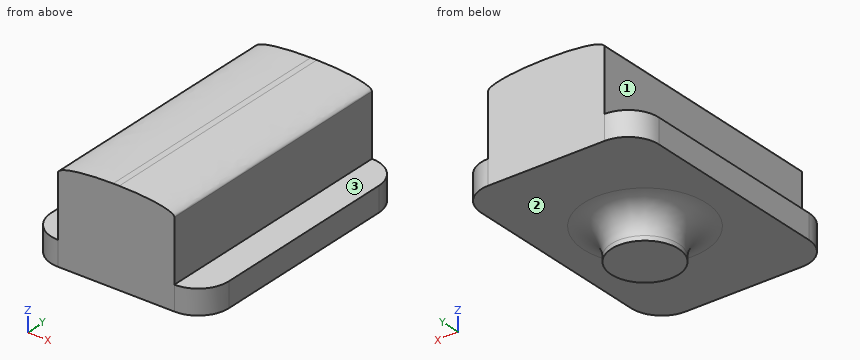
```python
from build123d import *

# Parameters (mm, degrees)
EXTRUDE_1_DEPTH          = 3.1
EXTRUDE_2_DEPTH          = 0.8
FILLET_1_SIZE            = 0.3
FILLET_1_SIZE_2          = 1.8
SKETCH_3_R               = 1
SKETCH_3_R_2             = 1.096749421
EXTRUDE_3_DEPTH          = 1.05
FILLET_5_R               = 0.9
CUT_EXTRUDE_2_DEPTH      = 82.307539193
CUT_EXTRUDE_2_DEPTH_BACK = 82.307539193
SKETCH_7_W               = 25.8
SKETCH_7_H               = 28.300000874
SKETCH_7_W_2             = 5.8
SKETCH_7_H_2             = 8.300000874
FILLET_6_R               = 1


with BuildPart() as part:
    # 草图1 → 凸台-拉伸1 (new body)
    with BuildSketch(Plane.XY):
        with BuildLine():
            Line((-1.3, -78.273), (-1.3, -61.672998253))
            ThreePointArc((-1.3, -61.672998253), (0.6, -59.772998253), (2.5, -61.672998253))
            Line((2.5, -61.672998253), (2.5, -78.273))
            ThreePointArc((2.5, -78.273), (0.6, -80.173), (-1.3, -78.273))
        make_face()
    extrude(amount=EXTRUDE_1_DEPTH)

    # 草图2 → 凸台-拉伸2 (add)
    with BuildSketch(Plane(origin=(0, 0, 0), x_dir=(-1, 0, 0), z_dir=(0, 0, -1))):
        with BuildLine():
            Line((2.3, -78.273), (2.3, -61.672998253))
            ThreePointArc((2.3, -61.672998253), (-0.6, -58.772998253), (-3.5, -61.672998253))
            Line((-3.5, -61.672998253), (-3.5, -78.273))
            ThreePointArc((-3.5, -78.273), (-0.6, -81.173), (2.3, -78.273))
        make_face()
    extrude(amount=-EXTRUDE_2_DEPTH)

    # 圆角1
    # an asymmetric fillet: 1.8, 0.3 mm, written as the material it takes off along each edge
    with BuildSketch(Plane(origin=(2.5, -61.672998253, 3.1), x_dir=(0, 0, -1), z_dir=(0, -1, 0)), Plane(origin=(-1.3, -78.273, 3.1), x_dir=(0, 0, -1), z_dir=(0, 1, 0))) as fillet_1_piece_1:
        with BuildLine():
            Bezier((FILLET_1_SIZE, 0), (0, 0), (0, -FILLET_1_SIZE_2), weights=[1, 0.707106781, 1])
            Line((0, -FILLET_1_SIZE_2), (0, 0))
            Line((0, 0), (FILLET_1_SIZE, 0))
        make_face()
    extrude(amount=16.600001747, mode=Mode.SUBTRACT)
    with BuildSketch(Plane(origin=(0.6, -61.672998253, 3.1), x_dir=(-1, 0, 0), z_dir=(0, -1, 0))) as fillet_1_piece_2:
        with BuildLine():
            Bezier((1.9, FILLET_1_SIZE), (1.9, 0), (1.9 - FILLET_1_SIZE_2, 0), weights=[1, 0.707106781, 1])
            Line((1.9 - FILLET_1_SIZE_2, 0), (1.9, 0))
            Line((1.9, 0), (1.9, FILLET_1_SIZE))
        make_face()
    revolve(axis=Axis((0.6, -61.672998253, 3.1), (0, 0, -1)), revolution_arc=180, mode=Mode.SUBTRACT)
    with BuildSketch(Plane(origin=(0.6, -78.273, 3.1), x_dir=(1, 0, 0), z_dir=(0, 1, 0))) as fillet_1_piece_3:
        with BuildLine():
            Bezier((1.9, FILLET_1_SIZE), (1.9, 0), (1.9 - FILLET_1_SIZE_2, 0), weights=[1, 0.707106781, 1])
            Line((1.9 - FILLET_1_SIZE_2, 0), (1.9, 0))
            Line((1.9, 0), (1.9, FILLET_1_SIZE))
        make_face()
    revolve(axis=Axis((0.6, -78.273, 3.1), (0, 0, -1)), revolution_arc=180, mode=Mode.SUBTRACT)

    # 草图3 → 凸台-拉伸3 (add)
    with BuildSketch(Plane(origin=(0, 0, 0), x_dir=(-1, 0, 0), z_dir=(0, 0, -1))):
        with Locations(Location((-0.6, -61.672998253, 0), (0, 0, 180))):
            Circle(SKETCH_3_R)
        with Locations(Location((-0.6, -69.972999126, 0), (0, 0, 180))):
            Circle(SKETCH_3_R_2)
        with Locations(Location((-0.6, -78.273, 0), (0, 0, 180))):
            Circle(SKETCH_3_R_2)
    extrude(amount=EXTRUDE_3_DEPTH)

    # 圆角5
    fillet_5_edges = [part.edges().sort_by_distance(p)[0] for p in [
        (-0.4, -61.672998253, 0),
        (-0.496749421, -69.972999126, 0),
        (-0.496749421, -78.273, 0),
    ]]
    fillet(fillet_5_edges, radius=FILLET_5_R)

    # 草图7 → 切除-拉伸2 (cut, two sides: drawn at the far end of the back side and taken through both)
    with BuildSketch(Plane(origin=(0, 0, 0), x_dir=(-1, 0, 0), z_dir=(0, 0, -1)).offset(-CUT_EXTRUDE_2_DEPTH_BACK)):
        with Locations((-0.6, -69.972999126)):
            Rectangle(SKETCH_7_W, SKETCH_7_H)
        with Locations((-0.6, -69.972999126)):
            Rectangle(SKETCH_7_W_2, SKETCH_7_H_2, mode=Mode.SUBTRACT)
    extrude(amount=CUT_EXTRUDE_2_DEPTH + CUT_EXTRUDE_2_DEPTH_BACK, mode=Mode.SUBTRACT)

    # 圆角6
    fillet_6_edges = [part.edges().sort_by_distance(p)[0] for p in [
        (3.5, -74.122999563, 0.4),
        (3.5, -65.822998689, 0.4),
        (-2.3, -65.822998689, 0.4),
        (-2.3, -74.122999563, 0.4),
    ]]
    fillet(fillet_6_edges, radius=FILLET_6_R)


solid = part.part
```
Build history of the part. All positions in model axes, mm. Face numbers are marked on the shaded views. A direction names the side the tool comes from. Coordinates: 2 decimals unless noted, no trailing zeros. Order: outer loops, then holes, each group sorted by start corner. A loop starts at its lowest first (then second) coordinate and runs counter-clockwise, first axis right, second up. Notation, with made-up numbers: (-15, 20.25) -> (35, 20.25) arc R24 cw to (35, 38.25) -> close; hole circle Ø5 at (-35, -12.5). An arc over 180 degrees is marked (long way). Answer in a Markdown table with one row per item. Add a question column.
Q1. Drop flat-ended pins along their axis: pin 1 (0.6 mm diameter, centred on y = -70.5, z = 2, fed in from +X); pin 2 (1 mm diameter, centred on y = -69.5, z = 1.5, fed in from -X). Give the stop position or say it passes through.
Q2. Band-saw the part on A-A, the plane x = 0.6. List the corners of the cut face in (y, z), then the cut area to 3 significant figures.
Q3. Wall check: line 1 along Z through (x, y) = (2.8, -70.25); line 2 along X through (y, z) = (-73.5, 2.6); line 3 along Z through (x, y) = (0.9, -69). Give the ranges that are in metal, low to high. Write a range as [from, to].
Q4. Band-saw the part on B-B, the plane z = 2.25. List the corners of the cut face in (x, y), then the cut area to 3 significant figures.
Q5. Which spindle directions (+Z, -Z, +X, -X, +Y, -Y) get a long thin tool onto all of the face, cutting with end or side? Do the marked faces 1, 2 and 3. Say none if no direction does.
Q6. Band-saw the part on C-C, the plane z = -0.1. List the corners of the cut face in (x, y).
Answers follow:
| question | item | result |
|---|---|---|
| 1 | pin 1 | x = 2.5 |
| 1 | pin 2 | x = -1.3 |
| 2 | outline | (-74.12, 0) -> (-71.97, 0) arc R0.9 cw to (-71.07, -0.9) -> (-71.07, -1.05) -> (-68.88, -1.05) -> (-68.88, -0.9) arc R0.9 cw to (-67.98, 0) -> (-65.82, 0) -> (-65.82, 3.1) -> (-74.12, 3.1) -> close |
| 2 | area | 28.4 mm^2 |
| 3 | line 1 | [0, 0.8] |
| 3 | line 2 | [-1.3, 2.5] |
| 3 | line 3 | [-1.05, 3.1] |
| 4 | outline | (-1.3, -74.12) -> (2.5, -74.12) -> (2.5, -65.82) -> (-1.3, -65.82) -> close |
| 4 | area | 31.5 mm^2 |
| 5 | face 1 | +Z, -X, +Y, -Y |
| 5 | face 2 | -Z |
| 5 | face 3 | +Z, +X, +Y, -Y |
| 6 | outline | circle Ø3.17 at (0.6, -69.97) |
